The listing builds one solid part. Answer for the finished solid, in the listing's coordinates (mm). A direction names the side the tool comes from. Round coordinates to 2 decimals unless told otherwise and drop trailing zeros. Write each loop counter-clockwise with the first axis right and the second up, starting at its lowest first coordinate (ties: lowest second). Pieces come first, ordered by that corner, then holes. Notation, with made-up numbers: (11, 25.5) - (26, 25.5) arc R31 cw to (26, 57.5) - close; hole circle Ø3 at (15.5, 46). An arc over 180 degrees is marked (long way). Answer as CSV lines item,"result". Start each with the question number.
Item 1: Which of the six approach directions +Z, -Z, +X, -X, +Y, -Y give full straight-line access (tool end or side, diameter ignored) to faces 1 (the flat face through (14.986, 19, 0)), 2 (the flat face through (-2.54, -1, 0)), 3 (the flat face through (-6, -1, -6.35)), 4 (the flat face through (-8.89, -1, 0))?
Item 2: A cutting plane is placed at D-D on z = -11.5. Determine the outline of the cut face in (x, y).
Item 3: A cutting plane is placed at C-C on y = 19.05. Determine the outline of the cut face in (x, z), and give its area (3 significant figures).
Item 4: For a pull along Z with two mould halves and no side action, classify faces 5 (the cylindrical face through (17.056, 19.281, -18.286)), 6 (the cylindrical face through (16.403, 33.777, 1.934)), 7 (the flat face through (17.78, 4, 0)) as pulls with the +Z half, pulls with the -Z half, needs draft (parallel to the pull), parting line crosses it, or undercut.
Item 5: Flat-ended cylindrical pins translate along their axes: pin 1 (1.5 mm diameter, centred on y = 21, z = -3, fed in from +X); pin 2 (0.6 mm diameter, centred on y = -0.5, z = -1, fed in from -X); pin 3 (3 mm diameter, centred on x = 13, z = -8, fed in from -Y). Find the tip coordinate at first contact, or state that the pin passes through.
Item 6: A cutting plane is placed at B-B on x = -14.5. Determine the outline of the cut face in (y, z), and give its area (3 significant figures).
Item 7: A cutting plane is placed at A-A on z = 0. Determine the outline of the cut face in (x, y), and give its area (3 significant figures).
Item 8: Straight lines are drawn through the part: line 1 along X through (y, z) = (33, -2); line 2 along Y through (x, z) = (-14, -16); line 3 along Y through (x, z) = (16, -2). For each, find the intervals that lie inside material, in ascending order. Write a range as [from, to].
```python
from build123d import *

# Parameters (mm, degrees)
SKETCH1_W           = 35.56
SKETCH1_H           = 38.1
BOSS_EXTRUDE1_DEPTH = 38.1
FILLET1_R           = 2.54
SKETCH4_R           = 14.853609937
CUT_EXTRUDE2_DEPTH  = 2.794
SKETCH5_W           = 6.35
SKETCH5_H           = 12.7
BOSS_EXTRUDE2_DEPTH = 1.27


with BuildPart() as part:
    # Sketch1 → Boss-Extrude1 (new body)
    with BuildSketch(Plane(origin=(0, 0, 0), x_dir=(1, 0, 0), z_dir=(0, 1, 0))):
        Rectangle(SKETCH1_W, SKETCH1_H)
    extrude(amount=BOSS_EXTRUDE1_DEPTH)

    # Fillet1
    fillet1_edges = [part.edges().sort_by_distance(p)[0] for p in [
        (-17.78, 38.1, 0),
        (0, 38.1, 19.05),
        (17.78, 38.1, 0),
        (0, 0, 19.05),
        (-17.78, 0, 0),
        (0, 0, -19.05),
        (17.78, 0, 0),
        (17.78, 19.05, 19.05),
        (-17.78, 19.05, 19.05),
        (-17.78, 19.05, -19.05),
        (17.78, 19.05, -19.05),
        (0, 38.1, -19.05),
    ]]
    fillet(fillet1_edges, radius=FILLET1_R)

    # Sketch4 → Cut-Extrude2 (cut)
    with BuildSketch(Plane(origin=(17.78, 0, 0), x_dir=(0, 0, -1), z_dir=(1, 0, 0))):
        with Locations((0, 19.05)):
            Circle(SKETCH4_R)
    extrude(amount=-CUT_EXTRUDE2_DEPTH, mode=Mode.SUBTRACT)

    # Sketch5 → Boss-Extrude2 (add)
    with BuildSketch(Plane.XZ):
        with Locations((-5.715, 0)):
            Rectangle(SKETCH5_W, SKETCH5_H)
    extrude(amount=BOSS_EXTRUDE2_DEPTH)


solid = part.part
```
Geometry says:
1,face 1,"+X"
1,face 2,"+Z, -Z, +X, -Y"
1,face 3,"-Z, +X, -X, -Y"
1,face 4,"+Z, -Z, -X, -Y"
2,outline,"(-17.78, 2.54) arc R2.54 ccw to (-15.24, 0) - (15.24, 0) arc R2.54 ccw to (17.78, 2.54) - (17.78, 9.65) - (14.99, 9.65) - (14.99, 28.45) - (17.78, 28.45) - (17.78, 35.56) arc R2.54 ccw to (15.24, 38.1) - (-15.24, 38.1) arc R2.54 ccw to (-17.78, 35.56) - close"
3,outline,"(-17.78, -16.51) arc R2.54 ccw to (-15.24, -19.05) - (15.24, -19.05) arc R2.54 ccw to (17.78, -16.51) - (17.78, -14.85) - (14.99, -14.85) - (14.99, 14.85) - (17.78, 14.85) - (17.78, 16.51) arc R2.54 ccw to (15.24, 19.05) - (-15.24, 19.05) arc R2.54 ccw to (-17.78, 16.51) - close"
3,area,"1,270 mm^2"
4,face 5,"pulls with the -Z half"
4,face 6,"undercut"
4,face 7,"needs draft"
5,pin 1,"stops at x = 14.99"
5,pin 2,"stops at x = -8.89"
5,pin 3,"stops at y = 0"
6,outline,"(0, -16.51) arc R2.54 ccw to (2.54, -19.05) - (35.56, -19.05) arc R2.54 ccw to (38.1, -16.51) - (38.1, 16.51) arc R2.54 ccw to (35.56, 19.05) - (2.54, 19.05) arc R2.54 ccw to (0, 16.51) - close"
6,area,"1,450 mm^2"
7,outline,"(-17.78, 2.54) arc R2.54 ccw to (-15.24, 0) - (-8.89, 0) - (-8.89, -1.27) - (-2.54, -1.27) - (-2.54, 0) - (15.24, 0) arc R2.54 ccw to (17.78, 2.54) - (17.78, 4.2) - (14.99, 4.2) - (14.99, 33.9) - (17.78, 33.9) - (17.78, 35.56) arc R2.54 ccw to (15.24, 38.1) - (-15.24, 38.1) arc R2.54 ccw to (-17.78, 35.56) - close"
7,area,"1,270 mm^2"
8,line 1,"x = [-17.78, 14.99]"
8,line 2,"y = [0, 38.1]"
8,line 3,"y = [0.12, 4.33], [33.77, 37.98]"
